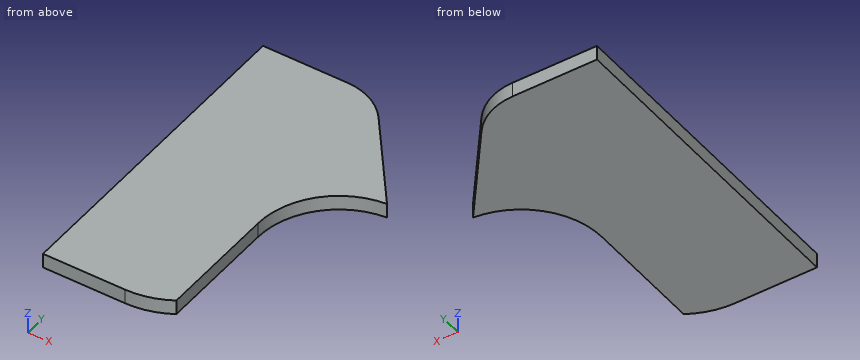
Autodesk Inventor part; units mm, degrees
ref_plane "Work Plane1" through (0, 0, -12.7) normal (0, 0, 1) x (1, 0, 0)
ref_plane "YZ Plane" through (0, 0, 0) normal (1, 0, 0) x (0, 1, 0)
ref_plane "XZ Plane" through (0, 0, 0) normal (0, 1, 0) x (-1, 0, 0)
ref_plane "Work Plane1" through (0, 0, -12.7) normal (0, 0, 1) x (1, 0, 0)
sketch "Sketch1" plane through (0, 0, -12.7) normal (0, 0, 1) x (1, 0, 0)
  line L0 (-47.625, 69.85) -> (-11.1125, 69.85)
  arc A0 (8.9541, 60.0222) -> (-11.1125, 69.85) centre (-11.1125, 44.45) ccw
  line L1 (8.9541, 60.0222) -> (38.3789, 22.1047)
  line L2 (-47.625, 69.85) -> (-47.625, -69.85)
  line L3 (-47.625, -69.85) -> (-12.2749, -69.85)
  arc A1 (-12.2749, -69.85) -> (9.777, -62.1413) centre (-12.2749, -34.4543) ccw
  line L4 (9.777, -62.1413) -> (30.2464, -45.838)
  arc A2 (38.3789, 22.1047) -> (30.2464, -45.838) centre (41.275, -12.7) ccw
  line L5 (56.3249, -1.0209) -> (8.9541, 60.0222) construction
  line L6 (-11.1125, 69.85) -> (-60.325, 69.85) construction
  line L7 (-60.325, -69.85) -> (-12.2749, -69.85) construction
  line L8 (9.777, -62.1413) -> (53.1434, -27.6012) construction
  circle A3 centre (41.275, -12.7) radius 9.525 construction
  line L9 (-60.325, 69.85) -> (-60.325, -69.85) construction
  circle A4 centre (-11.1125, 44.45) radius 10
  line L10 (6.35, -12.7) -> (6.35, -64.8708)
  line L11 (41.275, 22.225) -> (38.2856, 22.225)
  point P0 (0, 0)
  point P1 (16.8552, -56.5037)
  point P2 (38.2856, 22.225)
  point P3 (6.35, -64.5536)
  dimension "d0" = 12.7
  dimension "d1" = 34.925
  dimension "d4" = 20
extrude "Extrusion1" add sketch "Sketch1" along normal blind 6.35 contours L0 A0 L1 A2 L10 A1 L3 L2 | A4
properties part number "baseInner" material "Aluminum 6061"
Verification items for the finished model (mm, model axes). Give positions to 0.01 mm unless a question says otherwise; leave off trailing zeros. Loops run counter-clockwise (first coordinate to the right, second up) from the corner with the lowest first, then second, coordinate; pieces in that order, holes last.
1) Thickness scan on line 1 along X through (y, z) = (-47.5, -8) (3 decimals); line 2 along X through (y, z) = (50.5, -7) (3 decimals); line 3 along Y through (x, z) = (10, -10). Record the ranges inside material, lowest first.
2) Depth check by flat-ended pin: pin 1 Ø3 at (x, z) = (22, -10.5) entering from +Y; pin 2 Ø1.5 at (y, z) = (-26.5, -9) entering from +X. Enter the tip coordinate at first touch or a pass-through.
3) Sectioned sample at B-B, the plane x = 23. Enter the section's corners in (y, z).
4) Sectioned sample at C-C, the plane y = 40. Enter the section's corners in (x, z) (3 decimals), then the cut area to 3 significant figures.
Answers:
1. line 1: x = -47.625 to 6.35
1. line 2: x = -47.625 to 16.344
1. line 3: y = 2.84 to 58.67
2. pin 1: stops at y = 45.14
2. pin 2: stops at x = 6.35
3. outline: (17.06, -12.7) - (41.92, -12.7) - (41.92, -6.35) - (17.06, -6.35) - close
4. outline: (-47.625, -12.7) - (24.492, -12.7) - (24.492, -6.35) - (-47.625, -6.35) - close
4. area: 458 mm2
